```python
from build123d import *

# Parameters (mm, degrees)
F1_DEPTH      = 25.4
F3_DEPTH      = 25.4
F3_DEPTH_BACK = 50.801
F2_R          = 9.525
F4_DEPTH      = 25.4
F4_DEPTH_BACK = 50.801
F2_W          = 12.7
F2_H          = 2.54
F5_DEPTH      = 25.4
F5_DEPTH_BACK = 50.8
F7_DEPTH      = 25.4
F7_DEPTH_BACK = 50.801
F6_R          = 9.525
F8_DEPTH      = 25.4
F8_DEPTH_BACK = 50.801
F6_W          = 12.7
F6_H          = 2.54
F9_DEPTH      = 25.4
F9_DEPTH_BACK = 50.8


with BuildPart() as f1:
    # F0 (on Top) → F1 (new body)
    with BuildSketch(Plane.XY):
        Polygon((15.1580646015, 101.6), (-137.2419353985, 101.6), (-137.2419353985, 76.2), (-111.8419353985, 76.2), (-111.8419353985, 50.8), (-137.2419353985, 50.8), (-137.2419353985, 25.4), (-111.8419353985, 25.4), (-111.8419353985, 0), (40.5580646015, 0), (40.5580646015, 25.4), (15.1580646015, 25.4), (15.1580646015, 50.8), (40.5580646015, 50.8), (40.5580646015, 76.2), (15.1580646015, 76.2), align=None)
    extrude(amount=F1_DEPTH)

    # F2 (on face) → F3 (cut, two sides)
    with BuildSketch(Plane(origin=(0, 50.8, 0), x_dir=(-1, 0, 0), z_dir=(0, 1, 0))) as f3_sk:
        with BuildLine():
            ThreePointArc((124.5419353985, 22.86), (132.6241659074, 19.512230509), (135.9719353985, 11.43))
            ThreePointArc((135.9719353985, 11.43), (132.6241659074, 3.347769491), (124.5419353985, 0))
            Line((124.5419353985, 0), (137.2419353985, 0))
            Line((137.2419353985, 0), (137.2419353985, 25.4))
            Line((137.2419353985, 25.4), (124.5419353985, 25.4))
            Line((124.5419353985, 25.4), (124.5419353985, 22.86))
        make_face()
    extrude(amount=-F3_DEPTH, mode=Mode.SUBTRACT)
    extrude(f3_sk.sketch, amount=F3_DEPTH_BACK, mode=Mode.SUBTRACT)

    # F2 (on face) → F4 (cut, two sides)
    with BuildSketch(Plane(origin=(0, 50.8, 0), x_dir=(-1, 0, 0), z_dir=(0, 1, 0))) as f4_sk:
        with Locations((124.5419353985, 11.43)):
            Circle(F2_R)
    extrude(amount=-F4_DEPTH, mode=Mode.SUBTRACT)
    extrude(f4_sk.sketch, amount=F4_DEPTH_BACK, mode=Mode.SUBTRACT)

    # F2 (on face) → F5 (join, two sides)
    with BuildSketch(Plane(origin=(0, 50.8, 0), x_dir=(-1, 0, 0), z_dir=(0, 1, 0))) as f5_sk:
        with Locations((118.1919353985, 24.13)):
            Rectangle(F2_W, F2_H)
    extrude(amount=F5_DEPTH)
    extrude(f5_sk.sketch, amount=-F5_DEPTH_BACK)

    # F6 (on face) → F7 (cut, two sides)
    with BuildSketch(Plane.XZ.offset(-50.8)) as f7_sk:
        with BuildLine():
            ThreePointArc((27.8580646015, 22.86), (35.9402951105, 19.512230509), (39.2880646015, 11.43))
            ThreePointArc((39.2880646015, 11.43), (35.9402951105, 3.347769491), (27.8580646015, 0))
            Line((27.8580646015, 0), (40.5580646015, 0))
            Line((40.5580646015, 0), (40.5580646015, 25.4))
            Line((40.5580646015, 25.4), (27.8580646015, 25.4))
            Line((27.8580646015, 25.4), (27.8580646015, 22.86))
        make_face()
    extrude(amount=-F7_DEPTH, mode=Mode.SUBTRACT)
    extrude(f7_sk.sketch, amount=F7_DEPTH_BACK, mode=Mode.SUBTRACT)

    # F6 (on face) → F8 (cut, two sides)
    with BuildSketch(Plane.XZ.offset(-50.8)) as f8_sk:
        with Locations((27.8580646015, 11.43)):
            Circle(F6_R)
    extrude(amount=-F8_DEPTH, mode=Mode.SUBTRACT)
    extrude(f8_sk.sketch, amount=F8_DEPTH_BACK, mode=Mode.SUBTRACT)

    # F6 (on face) → F9 (join, two sides)
    with BuildSketch(Plane.XZ.offset(-50.8)) as f9_sk:
        with Locations((21.5080646015, 24.13)):
            Rectangle(F6_W, F6_H)
    extrude(amount=F9_DEPTH)
    extrude(f9_sk.sketch, amount=-F9_DEPTH_BACK)


solid = f1.part
```
For this review, take the finished solid that the model builds, in its own axes (mm). A direction names the side the tool comes from. Round coordinates to 2 decimals unless told otherwise and drop trailing zeros. Order: outer loops, then holes, each group sorted by start corner. A loop starts at its lowest first (then second) coordinate and runs counter-clockwise, first axis right, second up. Notation, with made-up numbers: (50.5, -17.75) -> (85.5, -17.75) arc R10 ccw to (85.5, -4.75) -> close; hole circle Ø10 at (60.5, 83). An arc over 180 degrees is marked (long way). Use a Markdown table: item, result.
Item 1: Machinability: for faces 1 (the flat face through (-111.842, 64, 11)), 2 (the flat face through (19, 76.2, 6)), 3 (the flat face through (-111.842, 13, 11)), 4 (the cylindrical face through (-133.627, 88.722, 14.291)), 5 (the flat face through (15.158, 38, 11)), which of the approach directions +Z, -Z, +X, -X, +Y, -Y give a long, thin tool a straight path to every point of the face, cutting with its end or side? Answer none if there is none.
Resolved:
| item | result |
|---|---|
| face 1 | -Z, -X |
| face 2 | -Z, +X, +Y |
| face 3 | -Z, -X, -Y |
| face 4 | +Y, -Y |
| face 5 | -Z, +X |
Item 2: For pin 1 (3 mm diameter, centred on y = 57.5, z = 24.5, fed in from -X); pin 2 (7 mm diameter, centred on y = 92, z = 10, fed in from +X); pin 3 (0.8 mm diameter, centred on y = 33.5, z = 23.5, fed in from +X); pin 4 (7 mm diameter, centred on x = 24, z = 11, fed in from +Y), all flat-tipped, find the tip position at first contact; note any pin that passes through.
Resolved:
| item | result |
|---|---|
| pin 1 | stops at x = -124.54 |
| pin 2 | stops at x = 15.16 |
| pin 3 | stops at x = 27.86 |
| pin 4 | passes through |
Item 3: Draft analysis for pull direction X (two halves, no side actions). For faces 6 (the cylindrical face through (26.618, 12.878, 20.874)), 7 (the flat face through (15.158, 89, 11)), 8 (the flat face through (-118, 63, 22.86)), state which applies: +X half, -X half, draft (parallel to the pull), parting line (faces both ways), or undercut.
Resolved:
| item | result |
|---|---|
| face 6 | undercut |
| face 7 | +X half |
| face 8 | draft |
Item 4: Take a section at A-A (y = 33). State the section outline as (x, z) points (3 decimals), plus the area to 3 significant figures.
Resolved:
| item | result |
|---|---|
| outline | (-124.542, 0) -> (15.158, 0) -> (15.158, 22.86) -> (27.858, 22.86) -> (27.858, 25.4) -> (-124.542, 25.4) -> (-124.542, 22.86) arc R11.43 ccw to start; hole circle Ø19.05 at (-124.542, 11.43) |
| area | 3,500 mm² |
Item 5: For line 1 along X through (y, z) = (13.5, 11.43); line 2 along Y through (x, z) = (-112, 15.5); line 3 along X through (y, z) = (84.75, 11.43), list the stretches that pass through material, from the lowest coordinate up. Write a range as [from, to].
Resolved:
| item | result |
|---|---|
| line 1 | x = [-111.84, 18.33], [37.38, 39.29] |
| line 2 | y = [25.4, 50.8], [76.2, 101.6] |
| line 3 | x = [-135.97, -134.07], [-115.02, 15.16] |
Item 6: Take a section at B-B (z = 9.75). State how many separate pieces and enclosed holes the cut face has, plus the area to 3 significant figures.
Resolved:
| item | result |
|---|---|
| separate pieces | 5 |
| enclosed holes | 0 |
| area | 13,400 mm² |
